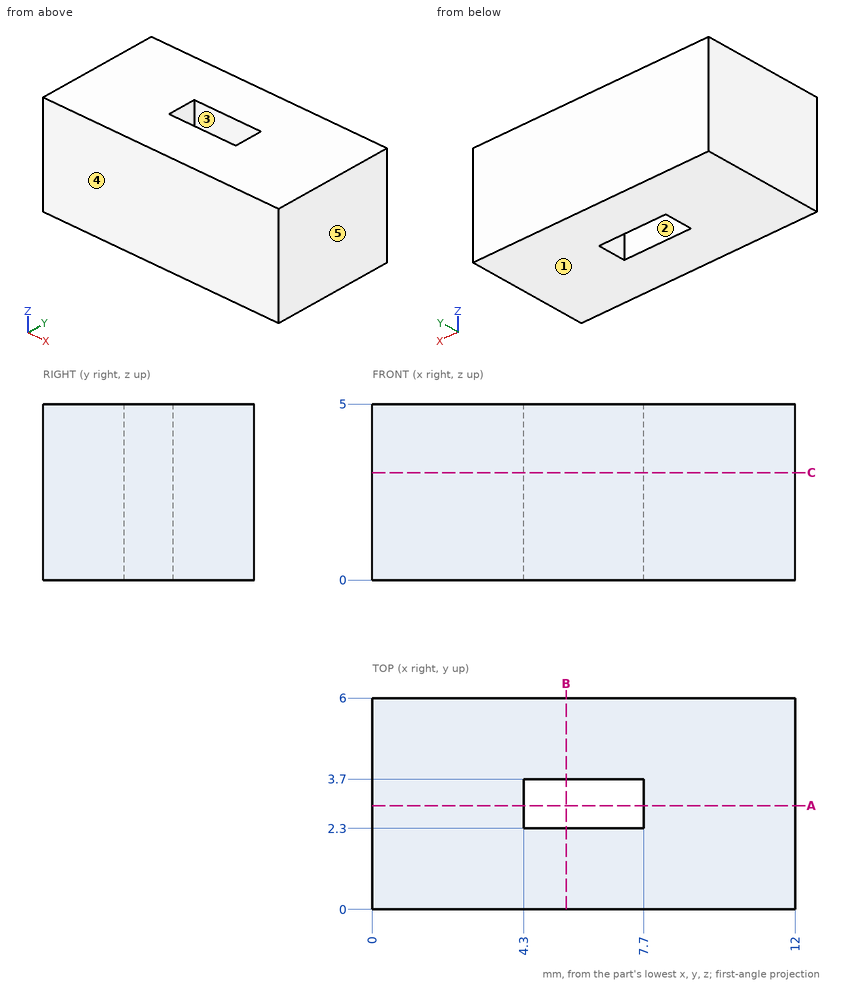
Job drawing, mm, ordinate dimensions from the low corner. One solid piece. A direction names the side the tool comes from. Give positions to 0.01 mm unless a question says otherwise; leave off trailing zeros. Order: outer loops, then holes, each group sorted by start corner. A loop starts at its lowest first (then second) coordinate and runs counter-clockwise, first axis right, second up. Notation, with made-up numbers: (88.5, 51.5) - (137.5, 51.5) arc R31 cw to (137.5, 77.5) - close; hole circle Ø3 at (83, 84.25). An arc over 180 degrees is marked (long way). One line per question, with ' | ' between items.
1. Band-saw the part on B-B on x = 5.5. List the corners of the cut face in (y, z).
Filled in:
outline: (0, 0) - (2.3, 0) - (2.3, 5) - (0, 5) - close; (3.7, 0) - (6, 0) - (6, 5) - (3.7, 5) - close
2. Which spindle directions (+Z, -Z, +X, -X, +Y, -Y) get a long thin tool onto all of the face, cutting with end or side? Do the marked faces 1 and 2. Say none if no direction does.
Filled in:
face 1: -Z, +X, -X, +Y, -Y | face 2: +Z, -Z
3. Drill centre lines: probe 1 along Y at (x, z) = (6.5, 4.35); probe 2 along X at (y, z) = (3, 2). Where is each one in solid material? Low to high.
Filled in:
probe 1: 0 to 2.3, 3.7 to 6 | probe 2: 0 to 4.3, 7.7 to 12
4. Band-saw the part on C-C on z = 3.05. List the corners of the cut face in (x, y).
Filled in:
outline: (0, 0) - (12, 0) - (12, 6) - (0, 6) - close; hole (4.3, 2.3) - (7.7, 2.3) - (7.7, 3.7) - (4.3, 3.7) - close
5. Pull direction Y, two halves, no side cores. Call the marked faces 3, 4 and 5: +Y half, -Y half, draft (parallel to the pull), parting line (faces both ways), or undercut.
Filled in:
face 3: undercut | face 4: -Y half | face 5: draft
6. Band-saw the part on A-A on y = 2.95. List the corners of the cut face in (x, z), then the cut area to 3 significant figures.
Filled in:
outline: (0, 0) - (4.3, 0) - (4.3, 5) - (0, 5) - close; (7.7, 0) - (12, 0) - (12, 5) - (7.7, 5) - close | area: 43.0 mm²
